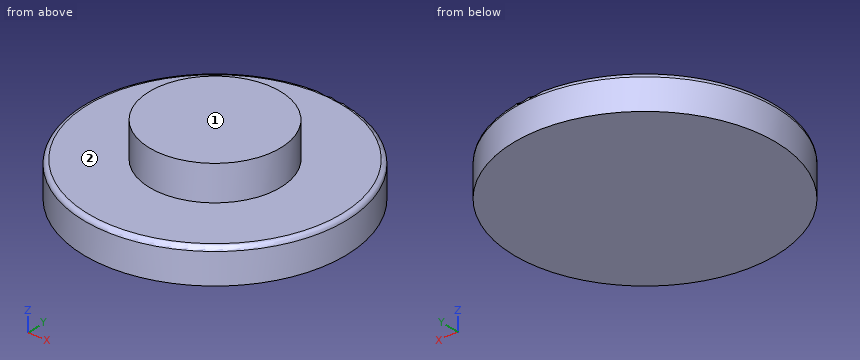
Autodesk Fusion 360 part; units mm, degrees
sketch "Sketch1" plane through (0, 0, 0) normal (0, 0, 1) x (1, 0, 0)
  circle A0 centre (0, 0) radius 150
extrude "Extrude1" add sketch "Sketch1" along normal blind 40
sketch "Sketch2" plane through (0, 0, 40) normal (0, 0, 1) x (-1, 0, 0)
  circle A0 centre (0, 0) radius 150
  circle A1 centre (0, 0) radius 75
extrude "Extrude2" add sketch "Sketch2" along normal blind 40 contours A1
fillet "Fillet1" radius 5 1 edges at (-139.8491, -54.2423, 40)
Can you work these out from the model? Positions are in its coordinate system, mm. Face numbers are marked on the shaded views. A direction names the side the tool comes from. Round coordinates to 2 decimals unless told otherwise and drop trailing zeros. Loops run counter-clockwise (first coordinate to the right, second up) from the corner with the lowest first, then second, coordinate; pieces in that order, holes last. Notation, with made-up numbers: (58, 70.5) - (89, 70.5) arc R26 cw to (89, 98.5) - close; hole circle Ø7 at (77.5, 61.25). An arc over 180 degrees is marked (long way). Use CSV: the item, a comma, the result in double quotes. Start each with the question number.
1) If we section it at A-A on x = 0: Write out the boundary of the cut face in (y, z), plus the area to 3 significant figures.
2) If we section it at C-C on z = 70: Write out the boundary of the cut face in (x, y), plus the area to 3 significant figures.
3) Please list where these lines run through material, in increasing order: probe 1 along Z at (x, y) = (52, 81); probe 2 along X at (y, z) = (4.5, 5); probe 3 along Y at (x, z) = (-46, 25). Write a range as [from, to].
4) If we section it at D-D on z = 28: Write out the boundary of the cut face in (x, y).
5) For the marked faces 1 and 2, which set-ups out of +Z, -Z, +X, -X, +Y, -Y let a thin tool reach every point of the face, with its end or its side?
6) For pin 1 Ø6 at (x, z) = (-60.5, 28) entering from -Y; pin 2 Ø1.5 at (y, z) = (-24.5, 42.5) entering from -X; pin 3 Ø6 at (x, z) = (-23.5, 52.5) entering from +Y, each with a flat end and sliding along its axis, tell me the tip position at first contact or that it passes through.
Geometry results:
1,outline,"(-150, 0) - (150, 0) - (150, 35) arc R5 ccw to (145, 40) - (75, 40) - (75, 80) - (-75, 80) - (-75, 40) - (-145, 40) arc R5 ccw to (-150, 35) - close"
1,area,"18,000 mm2"
2,outline,"circle Ø150 at (0, 0)"
2,area,"17,700 mm2"
3,probe 1,"z = [0, 40]"
3,probe 2,"x = [-149.93, 149.93]"
3,probe 3,"y = [-142.77, 142.77]"
4,outline,"circle Ø300 at (0, 0)"
5,face 1,"+Z, +X, -X, +Y, -Y"
5,face 2,"+Z"
6,pin 1,"stops at y = -138.54"
6,pin 2,"stops at x = -71.14"
6,pin 3,"stops at y = 72.14"
